Autodesk Inventor part; units mm, degrees
ref_plane "Work Plane1" through (40, 0, 0) normal (1, 0, 0) x (0, 0, -1)
ref_plane "YZ Plane" through (0, 0, 0) normal (1, 0, 0) x (0, 1, 0)
ref_plane "XZ Plane" through (0, 0, 0) normal (0, 1, 0) x (-1, 0, 0)
sketch "Sketch1" plane through (0, 0, 0) normal (1, 0, 0) x (0, 1, 0)
  line L0 (-15, 60) -> (15, 60)
  line L1 (15, 60) -> (15, -60)
  line L2 (15, -60) -> (-15, -60)
  line L3 (-15, -60) -> (-15, 60)
  line L4 (-15, 60) -> (15, -60) construction
  line L5 (15, 60) -> (-15, -60) construction
  point P0 (0, 0)
  dimension "d0" = 30
  dimension "d1" = 120
extrude "Extrusion1" add sketch "Sketch1" along normal blind 80
sketch "Sketch2" plane through (80, 0, 0) normal (1, 0, 0) x (0, 0, -1)
  line L0 (-60, 15) -> (-60, -15)
  line L1 (-60, 0) -> (60, 0)
  line L2 (60, -15) -> (60, 15)
  line L3 (60, 15) -> (-60, 15)
  line L4 (0, 15) -> (0, -15)
  line L5 (-60, -15) -> (60, -15)
  point P0 (0, 0)
  point P1 (-45, 0)
  point P2 (45, 0)
  dimension "d4" = 45
hole "Hole1" at (80, 0, 45) at (80, 0, -45) direction (-1, 0, 0) diameter 17.294 depth 41.2 tip angle 118
ref_plane "Work Plane1" through (40, 0, 0) normal (1, 0, 0) x (0, 0, -1)
mirror "Mirror1" about plane through (40, 0, 0) normal (1, 0, 0) of "Hole1"
sketch "Sketch5" plane through (0, 15, 60) normal (0, 1, 0) x (1, 0, 0)
  line L0 (0, 0) -> (80, 0)
  line L1 (40, 0) -> (40, 120)
  line L2 (0, 120) -> (80, 120)
  line L3 (55, 30) -> (25, 30)
  line L4 (25, 30) -> (25, 90)
  line L5 (25, 90) -> (55, 90)
  line L6 (55, 90) -> (55, 30)
  line L7 (55, 30) -> (25, 90) construction
  line L8 (25, 30) -> (55, 90) construction
  line L9 (0, 0) -> (0, 120)
  line L10 (0, 30) -> (10, 30)
  line L11 (10, 30) -> (10, 90)
  line L12 (10, 90) -> (0, 90)
  line L13 (0, 90) -> (0, 30)
  line L14 (80, 0) -> (80, 120)
  line L15 (80, 30) -> (70, 30)
  line L16 (70, 30) -> (70, 90)
  line L17 (70, 90) -> (80, 90)
  line L18 (80, 90) -> (80, 30)
  point P0 (0, 60)
  point P1 (40, 60)
  dimension "d20" = 30
  dimension "d22" = 30
  dimension "d23" = 30
  dimension "d24" = 60
  dimension "d25" = 10
  dimension "d26" = 10
extrude "Extrusion2" cut sketch "Sketch5" against normal through all contours L9 L12 L11 L10 | L3 L4 L5 L1 | L1 L5 L6 L3 | L15 L16 L17 L14
hole "Hole5" at (70, 0, 0) direction (-1, 0, 0) diameter 22 end through all
fillet "Fillet1" radius 2 4 edges at (40, 15, 60) (40, -15, 60) (40, -15, -60) (40, 15, -60)
fillet "Fillet4" radius 10 2 edges at (70, 0, 30) (10, 0, 30)
fillet "Fillet5" radius 5 2 edges at (25, 0, 30) (55, 0, 30)
fillet "Fillet6" radius 10 2 edges at (70, 0, -30) (10, 0, -30)
fillet "Fillet9" radius 5 2 edges at (25, 0, -30) (55, 0, -30)
properties part number "Profile_Middle_04"
Verification items for the finished model (mm, model axes). A direction names the side the tool comes from. Give positions to 0.01 mm unless a question says otherwise; leave off trailing zeros. Order: outer loops, then holes, each group sorted by start corner. A loop starts at its lowest first (then second) coordinate and runs counter-clockwise, first axis right, second up. Notation, with made-up numbers: (7, 1.25) - (11, 1.25) arc R8 cw to (11, 7.25) - close; hole circle Ø4 at (37, -32.75). An arc over 180 degrees is marked (long way). Answer as CSV lines item,"result". Start each with the question number.
Item 1: Section check C-C, the plane z = 0. Record the boundary of the cut face in (x, y).
Item 2: Gauge pin test, flat ends, axial feed: pin 1 (15 mm diameter, centred on y = 6, z = 3, fed in from +X); pin 2 (10 mm diameter, centred on y = 9, z = 17, fed in from +X); pin 3 (2 mm diameter, centred on y = -2.5, z = -39.5, fed in from -X). Record the tip position at first contact, or that the pin passes through.
Item 3: Material ranges on L1, parallel to Z at x = 15.25, y = 0; L2, parallel to Z at x = 33, y = 0; L3, parallel to Y at x = 18, z = 0, recorded low to high.
Item 4: Mould release check, pull along Y, two halves, no side actions. Record for faces 4 (the face through (40.56, -5.262, -38.138)), 5 (the face through (40.56, 2.597, 36.752)), 6 (the face through (27, 0, 29)), 7 (the face through (22, -15, -1)): released by +Y, released by -Y, zero draft, split by the parting line, or undercut.
Item 5: Section check A-A, the plane x = 33. Record the boundary of the cut face in (y, z).
Item 6: Access from +Z, -Z, +X, -X, +Y, -Y to the whole of each face (thin tool, end or side, straight path). Record for faces 1 (the face through (54, 0, 28)), 2 (the face through (7.15, -0.21, 26.99)), 3 (the face through (72.85, -0.21, -26.99)).
Item 7: Section check B-B, the plane z = 45. Record the boundary of the cut face in (x, y), plus the area to 3 significant figures.
Item 8: Section check D-D, the plane x = 57. Record the boundary of the cut face in (y, z).
Filled in:
1,outline,"(10, -15) - (25, -15) - (25, -11) - (10, -11) - close; (10, 11) - (25, 11) - (25, 15) - (10, 15) - close; (55, -15) - (70, -15) - (70, -11) - (55, -11) - close; (55, 11) - (70, 11) - (70, 15) - (55, 15) - close"
2,pin 1,"x = 70"
2,pin 2,"x = 70.2"
2,pin 3,"through"
3,L1,"-60 to -53.65, -36.35 to -11, 11 to 36.35, 53.65 to 60"
3,L2,"-60 to -53.65, -36.35 to -30, 30 to 36.35, 53.65 to 60"
3,L3,"-15 to -11, 11 to 15"
4,face 4,"undercut"
4,face 5,"undercut"
4,face 6,"zero draft"
4,face 7,"released by -Y"
5,outline,"(-15, -58) arc R2 ccw to (-13, -60) - (13, -60) arc R2 ccw to (15, -58) - (15, -30) - (-15, -30) - close; (-15, 30) - (15, 30) - (15, 58) arc R2 ccw to (13, 60) - (-13, 60) arc R2 ccw to (-15, 58) - close; hole circle Ø17.29 at (0, -45); hole circle Ø17.29 at (0, 45)"
6,face 1,"+Y, -Y"
6,face 2,"-X, +Y, -Y"
6,face 3,"+X, +Y, -Y"
7,outline,"(0, -15) - (80, -15) - (80, -8.65) - (0, -8.65) - close; (0, 8.65) - (80, 8.65) - (80, 15) - (0, 15) - close"
7,area,"1,020 mm^2"
8,outline,"(-15, -58) arc R2 ccw to (-13, -60) - (13, -60) arc R2 ccw to (15, -58) - (15, 58) arc R2 ccw to (13, 60) - (-13, 60) arc R2 ccw to (-15, 58) - close; hole circle Ø22 at (0, 0); hole circle Ø17.29 at (0, -45); hole circle Ø17.29 at (0, 45)"
